Source: CAD feature listing. Evaluate the final solid. Frame: model axes, mm. Give positions to 0.01 mm unless a question says otherwise; leave off trailing zeros. Write each loop counter-clockwise with the first axis right and the second up, starting at its lowest first coordinate (ties: lowest second). Pieces come first, ordered by that corner, then holes.
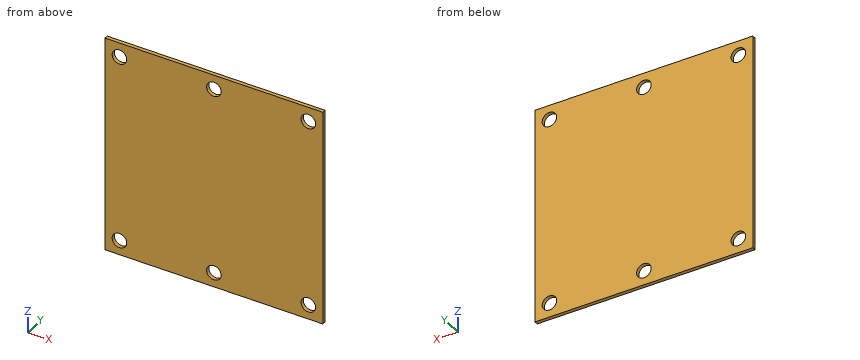
```python
from build123d import *

# Parameters (mm, degrees)
SKETCH1_W                    = 60
SKETCH1_H                    = 60
BOSS_EXTRUDE1_DEPTH          = 1
F_4_0_4_DIAMETER_HOLE1_D     = 4
F_4_0_4_DIAMETER_HOLE1_DEPTH = 1


with BuildPart() as part:
    # Sketch1 → Boss-Extrude1 (new body)
    with BuildSketch(Plane(origin=(0, 0, 0), x_dir=(1, 0, 0), z_dir=(0, 1, 0))):
        Rectangle(SKETCH1_W, SKETCH1_H)
    extrude(amount=BOSS_EXTRUDE1_DEPTH)

    # Ø4.0 (4) Diameter Hole1
    with Locations(Plane(origin=(0, 1, 0), x_dir=(1, 0, 0), z_dir=(0, 1, 0))):
        with Locations((26, 26), (0, 26), (-26, 26), (0, -26), (26, -26), (-26, -26)):
            Hole(F_4_0_4_DIAMETER_HOLE1_D / 2, depth=F_4_0_4_DIAMETER_HOLE1_DEPTH)


solid = part.part
```
1. Section query C-C (y = 0.8). Return loops of the section in (x, z), plus the area to 3 significant figures.
2. Section query D-D (x = 26.5). Return loops of the section in (y, z).
3. Section query B-B (z = -26). Return loops of the section in (x, y), plus the area to 3 significant figures.
4. Pin query (flat end, axial travel): P1, Ø3, axis at x = 26, z = 26, coming from the +Y side; P2, Ø6.5, axis at x = 0, z = 26, coming from the -Y side. Return the tip coordinate at first contact, or that it passes through.
5. Section query A-A (x = 0). Return loops of the section in (y, z), plus the area to 3 significant figures.
6. Line query: probe 1 along Z at (x, y) = (-26, 0.35); probe 2 along X at (y, z) = (0.7, -26); probe 3 along X at (y, z) = (0.3, -25). Output: solid intervals per line, ascending.
The answers:
1. outline: (-30, -30) - (30, -30) - (30, 30) - (-30, 30) - close; hole circle Ø4 at (-26, -26); hole circle Ø4 at (-26, 26); hole circle Ø4 at (0, -26); hole circle Ø4 at (0, 26); hole circle Ø4 at (26, -26); hole circle Ø4 at (26, 26)
1. area: 3,520 mm2
2. outline: (0, -30) - (1, -30) - (1, -27.94) - (0, -27.94) - close; (0, -24.06) - (1, -24.06) - (1, 24.06) - (0, 24.06) - close; (0, 27.94) - (1, 27.94) - (1, 30) - (0, 30) - close
3. outline: (-30, 0) - (-28, 0) - (-28, 1) - (-30, 1) - close; (-24, 0) - (-2, 0) - (-2, 1) - (-24, 1) - close; (2, 0) - (24, 0) - (24, 1) - (2, 1) - close; (28, 0) - (30, 0) - (30, 1) - (28, 1) - close
3. area: 48.0 mm2
4. P1: passes through
4. P2: stops at y = 0
5. outline: (0, -30) - (1, -30) - (1, -28) - (0, -28) - close; (0, -24) - (1, -24) - (1, 24) - (0, 24) - close; (0, 28) - (1, 28) - (1, 30) - (0, 30) - close
5. area: 52.0 mm2
6. probe 1: z = -30 to -28, -24 to 24, 28 to 30
6. probe 2: x = -30 to -28, -24 to -2, 2 to 24, 28 to 30
6. probe 3: x = -30 to -27.73, -24.27 to -1.73, 1.73 to 24.27, 27.73 to 30
